Can you work these out from the drawing? Everything is in mm from the part's minimum corner. Coordinates: 2 decimals unless noted, no trailing zeros. Order: outer loops, then holes, each group sorted by start corner. A loop starts at its lowest first (then second) coordinate and runs counter-clockwise, first axis right, second up. Notation, with made-up numbers: M -26,68.5 L -5,68.5 A27 ccw -5,91.5 Z; hole C -7.5,69 d11. An arc over 180 degrees is marked long. Answer as a JSON object with one key per item and string values.
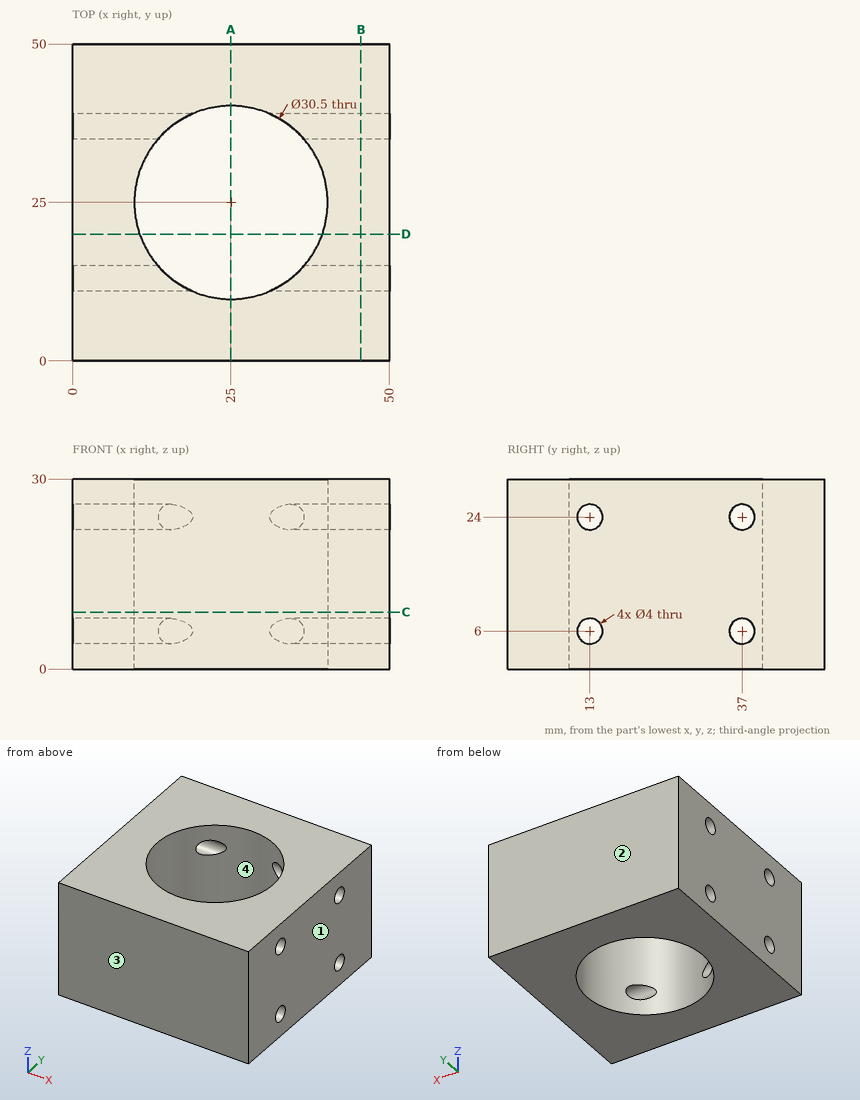
Item 1: If we mould it in two halves opening along Y, with no side actions, what happens to the marked faces 1, 2, 3 and 4? For each: pulls with the +Y half, pulls with the -Y half, needs draft (parallel to the pull), parting line crosses it, or undercut.
Answers follow:
{"face 1": "needs draft", "face 2": "pulls with the +Y half", "face 3": "pulls with the -Y half", "face 4": "undercut"}
Item 2: I want a section at C-C, the plane z = 9. Write out the boundary of the cut face in (x, y).
Answers follow:
{"outline": "M 0,0 L 50,0 L 50,50 L 0,50 Z; hole C 25,25 d30.5"}
Item 3: I'm going to push flat-ended pins straight in: pin 1 (6.5 mm diameter, centred on y = 13, z = 6, fed in from +X); pin 2 (1 mm diameter, centred on x = 25.5, y = 38, fed in from -Z). Where does each tip first touch, or does it pass through?
Answers follow:
{"pin 1": "stops at x = 50", "pin 2": "passes through"}
Item 4: I want a section at D-D, the plane y = 20. Write out the boundary of the cut face in (x, z).
Answers follow:
{"outline": "M 0,0 L 10.59,0 L 10.59,30 L 0,30 Z; M 39.41,0 L 50,0 L 50,30 L 39.41,30 Z"}
Item 5: I want a section at A-A, the plane x = 25. Write out the boundary of the cut face in (y, z).
Answers follow:
{"outline": "M 0,0 L 9.75,0 L 9.75,30 L 0,30 Z; M 40.25,0 L 50,0 L 50,30 L 40.25,30 Z"}
Item 6: I want a section at B-B, the plane x = 45.5. Write out the boundary of the cut face in (y, z).
Answers follow:
{"outline": "M 0,0 L 50,0 L 50,30 L 0,30 Z; hole C 13,6 d4; hole C 13,24 d4; hole C 37,6 d4; hole C 37,24 d4"}
Item 7: Please list where these lines run through material, in increasing order: line 1 (Z direction, x = 40.25, y = 13); line 2 (Y direction, x = 4, z = 25); line 3 (Y direction, x = 25, z = 23).
Answers follow:
{"line 1": "z = 0 to 4, 8 to 22, 26 to 30", "line 2": "y = 0 to 11.27, 14.73 to 35.27, 38.73 to 50", "line 3": "y = 0 to 9.75, 40.25 to 50"}
